Geometry check sheet. Reference: drawing and pictorial views, mm from the part's lowest x, y, z. Coordinates: 2 decimals unless noted, no trailing zeros. Order: outer loops, then holes, each group sorted by start corner. A loop starts at its lowest first (then second) coordinate and runs counter-clockwise, first axis right, second up. Notation, with made-up numbers: M 42,32 L 62,32 A16 cw 62,43 Z; hole C 42,73.25 d4. An arc over 180 degrees is marked long. Return JSON: item names as keys, results as strings.
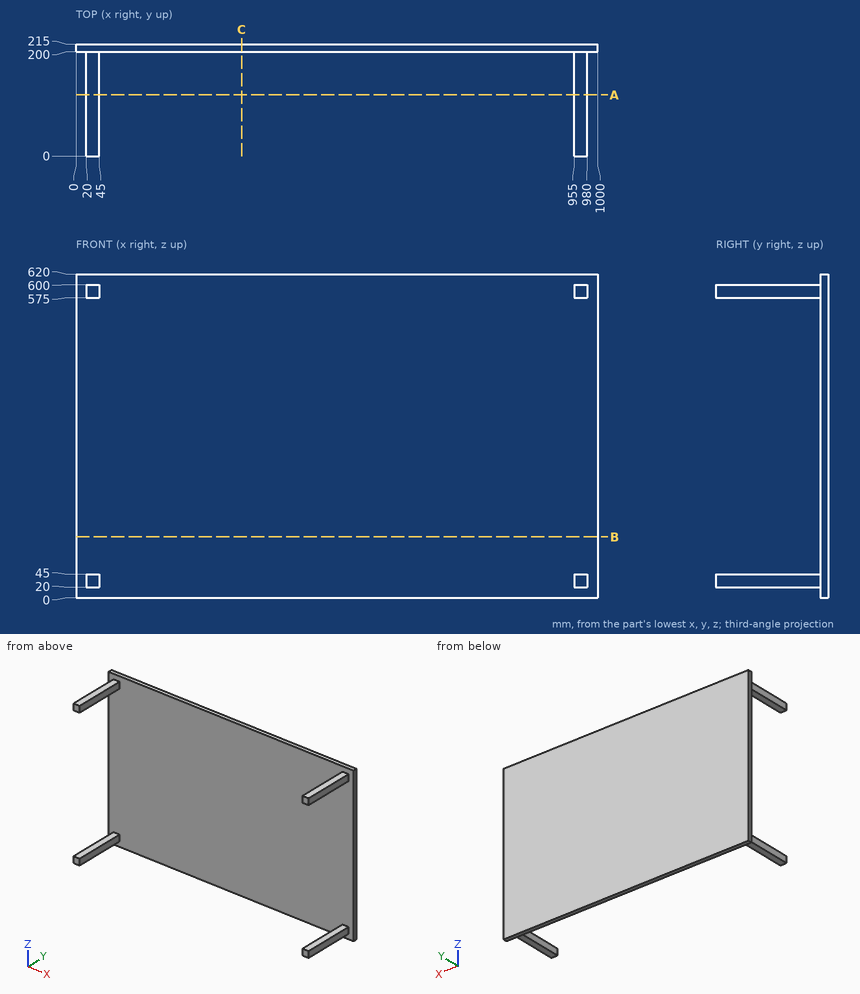
Q1. Cross-section at A-A, the plane y = 117.5. Record the boundary of the cut face in (x, z).
Values:
{"outline": "M 20,20 L 45,20 L 45,45 L 20,45 Z; M 20,575 L 45,575 L 45,600 L 20,600 Z; M 955,20 L 980,20 L 980,45 L 955,45 Z; M 955,575 L 980,575 L 980,600 L 955,600 Z"}
Q2. Cross-section at C-C, the plane x = 317.5. Record the boundary of the cut face in (y, z).
Values:
{"outline": "M 200,0 L 215,0 L 215,620 L 200,620 Z"}
Q3. Material ranges on line 1 along Y through (x, z) = (442, 517), recorded low to high.
Values:
{"line 1": "200 to 215"}
Q4. Cross-section at B-B, the plane z = 116.5. Record the boundary of the cut face in (x, y), and give its area (3 significant figures).
Values:
{"outline": "M 0,200 L 1000,200 L 1000,215 L 0,215 Z", "area": "15,000 mm^2"}
Q5. Go/stop test with flat-tipped pins: pin 1 (10 mm diameter, centred on x = 229.5, z = 261.5, fed in from -Y); pin 2 (12.5 mm diameter, centred on x = 965.5, y = 69.5, fed in from +Z); pin 3 (20 mm diameter, centred on y = 90.5, z = 586.5, fed in from +X). Record where each tip stops, or that it passes through.
Values:
{"pin 1": "y = 200", "pin 2": "z = 600", "pin 3": "x = 980"}
